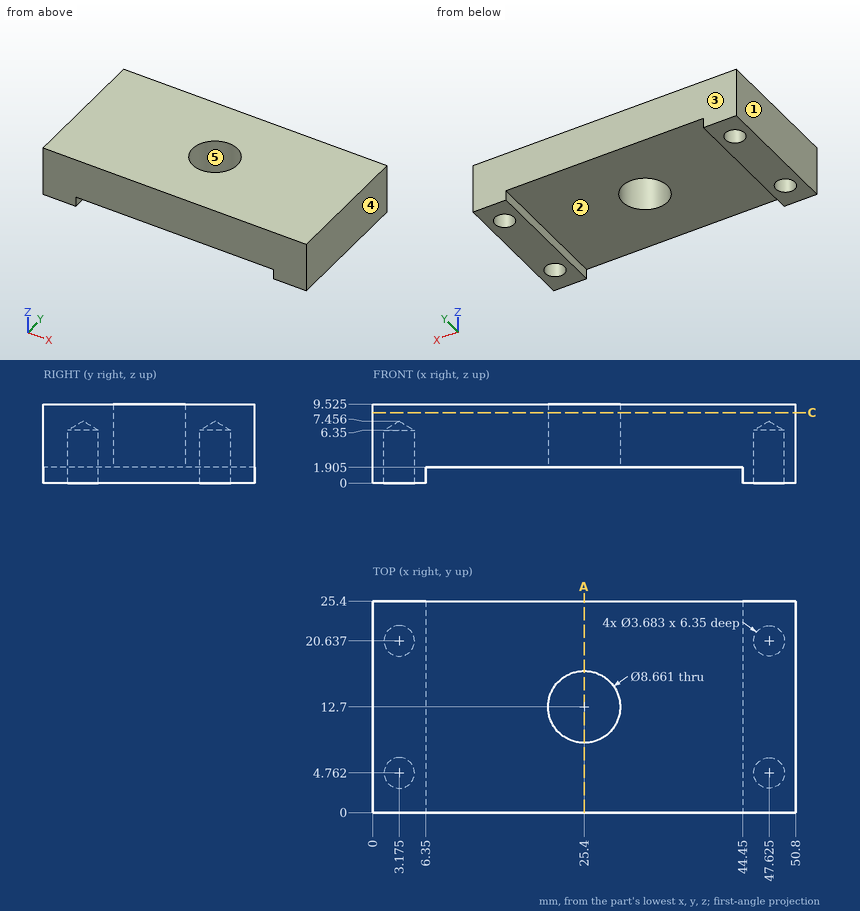
Print and shaded views of the part. All mm, measured from the part's lowest x, y and z. A direction names the side the tool comes from. Coordinates: 2 decimals unless noted, no trailing zeros. Order: outer loops, then holes, each group sorted by start corner. A loop starts at its lowest first (then second) coordinate and runs counter-clockwise, first axis right, second up. Notation, with made-up numbers: (10.25, 19.5) - (32.25, 19.5) arc R18 ccw to (32.25, 23.5) - close; hole circle Ø1 at (63.5, -19). An arc over 180 degrees is marked (long way). Return JSON: item names as keys, results as strings. Group by question number.
Item 1: Which spindle directions (+Z, -Z, +X, -X, +Y, -Y) get a long thin tool onto all of the face, cutting with end or side? Do the marked faces 1 and 2. Say none if no direction does.
Item 2: Pin check, flat tips, straight feed: pin 1 (8 mm diameter, centred on x = 25.4, y = 12.7, fed in from -Z); pin 2 (7.5 mm diameter, centred on x = 26.5, y = 11, fed in from -Z) (1 decimal); pin 3 (3 mm diameter, centred on x = 47.62, y = 20.64, fed in from -Z). Stop position of each tip, or through.
Item 3: Drill centre lines: probe 1 along X at (y, z) = (16, 1); probe 2 along X at (y, z) = (12.7, 5.75); probe 3 along X at (y, z) = (19.5, 6.25) (1 decimal). Where is each one in solid material? Low to high. Write a range as from..to.
Item 4: Pull direction X, two halves, no side cores. Call the marked faces 3, 4 and 5: pulls with the +X half, pulls with the -X half, needs draft (parallel to the pull), parting line crosses it, or undercut.
Item 5: Cut at A-A (x = 25.4). List the corners of the cut face in (y, z) (1 decimal).
Item 6: Cut at C-C (z = 8.5). List the corners of the cut face in (x, y).
Check values:
{
 "1": {"face 1": "+Z, -Z, -X, +Y, -Y", "face 2": "-Z, +Y, -Y"},
 "2": {"pin 1": "passes through", "pin 2": "stops at z = 1.9", "pin 3": "stops at z = 6.55"},
 "3": {"probe 1": "x = 0..6.35, 44.45..50.8", "probe 2": "x = 0..21.07, 29.73..50.8", "probe 3": "x = 0..1.7, 4.6..46.2, 49.1..50.8"},
 "4": {"face 3": "needs draft", "face 4": "pulls with the +X half", "face 5": "undercut"},
 "5": {"outline": "(0, 1.9) - (8.4, 1.9) - (8.4, 9.5) - (0, 9.5) - close; (17, 1.9) - (25.4, 1.9) - (25.4, 9.5) - (17, 9.5) - close"},
 "6": {"outline": "(0, 0) - (50.8, 0) - (50.8, 25.4) - (0, 25.4) - close; hole circle Ø8.66 at (25.4, 12.7)"}
}
